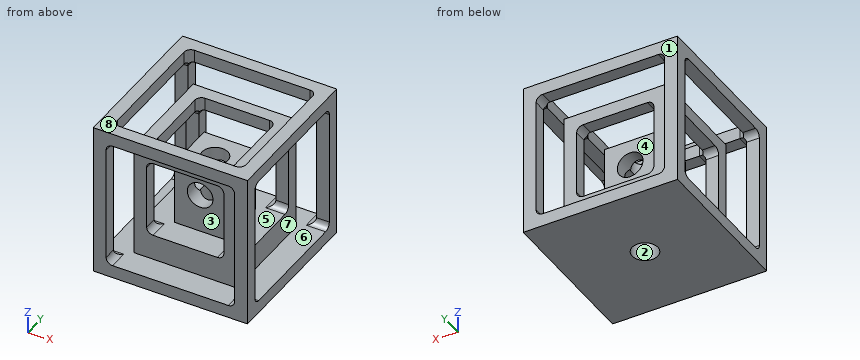
from build123d import *

# Parameters (mm, degrees)
SKETCH1_W           = 152.4
SKETCH1_H           = 152.4
EXTRUDE2_DEPTH      = 152.4
CUT_EXTRUDE14_DEPTH = 25.4
CUT_EXTRUDE18_DEPTH = 25.4
CUT_EXTRUDE19_DEPTH = 25.4
CUT_EXTRUDE21_START = -25.4
CUT_EXTRUDE21_DEPTH = 25.4
CUT_EXTRUDE22_START = -25.4
CUT_EXTRUDE22_DEPTH = 25.4
CUT_EXTRUDE24_DEPTH = 25.4
CUT_EXTRUDE27_DEPTH = 25.4
CUT_EXTRUDE28_START = -25.4
CUT_EXTRUDE28_DEPTH = 25.4
CUT_EXTRUDE29_DEPTH = 25.4
CUT_EXTRUDE30_START = -25.4
CUT_EXTRUDE30_DEPTH = 25.4
SKETCH30_R          = 12.7
CUT_EXTRUDE31_DEPTH = 239.273120599
SKETCH31_R          = 12.7
CUT_EXTRUDE32_DEPTH = 239.273120599
SKETCH32_R          = 12.7
CUT_EXTRUDE33_DEPTH = 239.273120599
SCALE1_SCALE        = 2


with BuildPart() as part:
    # Sketch1 → Extrude2 (new body)
    with BuildSketch(Plane(origin=(0, 0, 0), x_dir=(1, 0, 0), z_dir=(0, 1, 0))):
        with Locations((76.2, 76.2)):
            Rectangle(SKETCH1_W, SKETCH1_H)
    extrude(amount=EXTRUDE2_DEPTH)

    # Sketch13 → Cut-Extrude14 (cut)
    with BuildSketch(Plane(origin=(0, 152.4, 0), x_dir=(1, 0, 0), z_dir=(0, 1, 0))):
        with BuildLine():
            Line((19.05, 12.7), (133.35, 12.7))
            ThreePointArc((133.35, 12.7), (137.840128061, 14.559871939), (139.7, 19.05))
            Line((139.7, 19.05), (139.7, 133.35))
            ThreePointArc((139.7, 133.35), (137.840128061, 137.840128061), (133.35, 139.7))
            Line((133.35, 139.7), (19.05, 139.7))
            ThreePointArc((19.05, 139.7), (14.559871939, 137.840128061), (12.7, 133.35))
            Line((12.7, 133.35), (12.7, 19.05))
            ThreePointArc((12.7, 19.05), (14.559871939, 14.559871939), (19.05, 12.7))
        make_face()
    extrude(amount=-CUT_EXTRUDE14_DEPTH, mode=Mode.SUBTRACT)

    # Sketch17 → Cut-Extrude18 (cut)
    with BuildSketch(Plane.XY):
        with BuildLine():
            Line((19.05, 12.7), (133.35, 12.7))
            ThreePointArc((133.35, 12.7), (137.840128061, 14.559871939), (139.7, 19.05))
            Line((139.7, 19.05), (139.7, 133.35))
            ThreePointArc((139.7, 133.35), (137.840128061, 137.840128061), (133.35, 139.7))
            Line((133.35, 139.7), (19.05, 139.7))
            ThreePointArc((19.05, 139.7), (14.559871939, 137.840128061), (12.7, 133.35))
            Line((12.7, 133.35), (12.7, 19.05))
            ThreePointArc((12.7, 19.05), (14.559871939, 14.559871939), (19.05, 12.7))
        make_face()
    extrude(amount=-CUT_EXTRUDE18_DEPTH, mode=Mode.SUBTRACT)

    # Sketch18 → Cut-Extrude19 (cut)
    with BuildSketch(Plane(origin=(152.4, 0, 0), x_dir=(0, 0, -1), z_dir=(1, 0, 0))):
        with BuildLine():
            Line((19.05, 12.7), (133.35, 12.7))
            ThreePointArc((133.35, 12.7), (137.840128061, 14.559871939), (139.7, 19.05))
            Line((139.7, 19.05), (139.7, 133.35))
            ThreePointArc((139.7, 133.35), (137.840128061, 137.840128061), (133.35, 139.7))
            Line((133.35, 139.7), (19.05, 139.7))
            ThreePointArc((19.05, 139.7), (14.559871939, 137.840128061), (12.7, 133.35))
            Line((12.7, 133.35), (12.7, 19.05))
            ThreePointArc((12.7, 19.05), (14.559871939, 14.559871939), (19.05, 12.7))
        make_face()
    extrude(amount=-CUT_EXTRUDE19_DEPTH, mode=Mode.SUBTRACT)

    # Sketch20 → Cut-Extrude21 (cut)
    with BuildSketch(Plane.ZY.offset(CUT_EXTRUDE21_START)):
        with BuildLine():
            Line((-133.35, 12.7), (-19.05, 12.7))
            ThreePointArc((-19.05, 12.7), (-14.559871939, 14.559871939), (-12.7, 19.05))
            Line((-12.7, 19.05), (-12.7, 133.35))
            ThreePointArc((-12.7, 133.35), (-14.559871939, 137.840128061), (-19.05, 139.7))
            Line((-19.05, 139.7), (-133.35, 139.7))
            ThreePointArc((-133.35, 139.7), (-137.840128061, 137.840128061), (-139.7, 133.35))
            Line((-139.7, 133.35), (-139.7, 19.05))
            ThreePointArc((-139.7, 19.05), (-137.840128061, 14.559871939), (-133.35, 12.7))
        make_face()
    extrude(amount=CUT_EXTRUDE21_DEPTH, mode=Mode.SUBTRACT)

    # Sketch21 → Cut-Extrude22 (cut)
    with BuildSketch(Plane.XZ.offset(CUT_EXTRUDE22_START)):
        with BuildLine():
            Line((19.05, -139.7), (133.35, -139.7))
            ThreePointArc((133.35, -139.7), (137.840128061, -137.840128061), (139.7, -133.35))
            Line((139.7, -133.35), (139.7, -19.05))
            ThreePointArc((139.7, -19.05), (137.840128061, -14.559871939), (133.35, -12.7))
            Line((133.35, -12.7), (19.05, -12.7))
            ThreePointArc((19.05, -12.7), (14.559871939, -14.559871939), (12.7, -19.05))
            Line((12.7, -19.05), (12.7, -133.35))
            ThreePointArc((12.7, -133.35), (14.559871939, -137.840128061), (19.05, -139.7))
        make_face()
    extrude(amount=CUT_EXTRUDE22_DEPTH, mode=Mode.SUBTRACT)

    # Sketch23 → Cut-Extrude24 (cut)
    with BuildSketch(Plane.XY.offset(-25.4)):
        with BuildLine():
            Line((44.45, 38.1), (107.95, 38.1))
            ThreePointArc((107.95, 38.1), (112.440128061, 39.959871939), (114.3, 44.45))
            Line((114.3, 44.45), (114.3, 107.95))
            ThreePointArc((114.3, 107.95), (112.440128061, 112.440128061), (107.95, 114.3))
            Line((107.95, 114.3), (44.45, 114.3))
            ThreePointArc((44.45, 114.3), (39.959871939, 112.440128061), (38.1, 107.95))
            Line((38.1, 107.95), (38.1, 44.45))
            ThreePointArc((38.1, 44.45), (39.959871939, 39.959871939), (44.45, 38.1))
        make_face()
    extrude(amount=-CUT_EXTRUDE24_DEPTH, mode=Mode.SUBTRACT)

    # Sketch26 → Cut-Extrude27 (cut)
    with BuildSketch(Plane.XZ.offset(-25.4)):
        with BuildLine():
            Line((44.45, -114.3), (107.95, -114.3))
            ThreePointArc((107.95, -114.3), (112.440128061, -112.440128061), (114.3, -107.95))
            Line((114.3, -107.95), (114.3, -44.45))
            ThreePointArc((114.3, -44.45), (112.440128061, -39.959871939), (107.95, -38.1))
            Line((107.95, -38.1), (44.45, -38.1))
            ThreePointArc((44.45, -38.1), (39.959871939, -39.959871939), (38.1, -44.45))
            Line((38.1, -44.45), (38.1, -107.95))
            ThreePointArc((38.1, -107.95), (39.959871939, -112.440128061), (44.45, -114.3))
        make_face()
    extrude(amount=-CUT_EXTRUDE27_DEPTH, mode=Mode.SUBTRACT)

    # Sketch27 → Cut-Extrude28 (cut)
    with BuildSketch(Plane(origin=(0, 127, 0), x_dir=(-1, 0, 0), z_dir=(0, 1, 0)).offset(CUT_EXTRUDE28_START)):
        with BuildLine():
            Line((-107.95, -114.3), (-44.45, -114.3))
            ThreePointArc((-44.45, -114.3), (-39.959871939, -112.440128061), (-38.1, -107.95))
            Line((-38.1, -107.95), (-38.1, -44.45))
            ThreePointArc((-38.1, -44.45), (-39.959871939, -39.959871939), (-44.45, -38.1))
            Line((-44.45, -38.1), (-107.95, -38.1))
            ThreePointArc((-107.95, -38.1), (-112.440128061, -39.959871939), (-114.3, -44.45))
            Line((-114.3, -44.45), (-114.3, -107.95))
            ThreePointArc((-114.3, -107.95), (-112.440128061, -112.440128061), (-107.95, -114.3))
        make_face()
    extrude(amount=CUT_EXTRUDE28_DEPTH, mode=Mode.SUBTRACT)

    # Sketch28 → Cut-Extrude29 (cut)
    with BuildSketch(Plane(origin=(25.4, 0, 0), x_dir=(0, -1, 0), z_dir=(-1, 0, 0))):
        with BuildLine():
            Line((-107.95, -114.3), (-44.45, -114.3))
            ThreePointArc((-44.45, -114.3), (-39.959871939, -112.440128061), (-38.1, -107.95))
            Line((-38.1, -107.95), (-38.1, -44.45))
            ThreePointArc((-38.1, -44.45), (-39.959871939, -39.959871939), (-44.45, -38.1))
            Line((-44.45, -38.1), (-107.95, -38.1))
            ThreePointArc((-107.95, -38.1), (-112.440128061, -39.959871939), (-114.3, -44.45))
            Line((-114.3, -44.45), (-114.3, -107.95))
            ThreePointArc((-114.3, -107.95), (-112.440128061, -112.440128061), (-107.95, -114.3))
        make_face()
    extrude(amount=-CUT_EXTRUDE29_DEPTH, mode=Mode.SUBTRACT)

    # Sketch29 → Cut-Extrude30 (cut)
    with BuildSketch(Plane.YZ.offset(127).offset(CUT_EXTRUDE30_START)):
        with BuildLine():
            Line((44.45, -114.3), (107.95, -114.3))
            ThreePointArc((107.95, -114.3), (112.440128061, -112.440128061), (114.3, -107.95))
            Line((114.3, -107.95), (114.3, -44.45))
            ThreePointArc((114.3, -44.45), (112.440128061, -39.959871939), (107.95, -38.1))
            Line((107.95, -38.1), (44.45, -38.1))
            ThreePointArc((44.45, -38.1), (39.959871939, -39.959871939), (38.1, -44.45))
            Line((38.1, -44.45), (38.1, -107.95))
            ThreePointArc((38.1, -107.95), (39.959871939, -112.440128061), (44.45, -114.3))
        make_face()
    extrude(amount=CUT_EXTRUDE30_DEPTH, mode=Mode.SUBTRACT)

    # Sketch30 → Cut-Extrude31 (cut, through all)
    with BuildSketch(Plane.XY.offset(-50.8)):
        with Locations((76.2, 76.2)):
            Circle(SKETCH30_R)
    extrude(amount=-CUT_EXTRUDE31_DEPTH, mode=Mode.SUBTRACT)

    # Sketch31 → Cut-Extrude32 (cut, through all)
    with BuildSketch(Plane(origin=(101.6, 0, 0), x_dir=(0, 0, -1), z_dir=(1, 0, 0))):
        with Locations((76.2, 76.2)):
            Circle(SKETCH31_R)
    extrude(amount=-CUT_EXTRUDE32_DEPTH, mode=Mode.SUBTRACT)

    # Sketch32 → Cut-Extrude33 (cut, through all)
    with BuildSketch(Plane.XZ.offset(-50.8)):
        with Locations(Location((76.2, -76.2, 0), (0, 0, 225))):
            Circle(SKETCH32_R)
    extrude(amount=-CUT_EXTRUDE33_DEPTH, mode=Mode.SUBTRACT)


with BuildPart() as part_1:
    # Scale1: scaled about (76.199999991, 76.199999991, -102.985994001)
    add(part.part.scale(SCALE1_SCALE).moved(Location((-76.199999991, -76.199999991, 102.985994001))))


solid = part_1.part
Can you work these out from the model? Positions are in its coordinate system, mm. Face numbers are marked on the shaded views. A direction names the side the tool comes from. Give positions to 0.01 mm unless a question says otherwise; leave off trailing zeros. Loops run counter-clockwise (first coordinate to the right, second up) from the corner with the lowest first, then second, coordinate; pieces in that order, holes last. Notation, with made-up numbers: (77, 81) - (106, 81) arc R23 cw to (106, 119) - close; hole circle Ø7 at (88, 5.5). An arc over 180 degrees is marked (long way). Return JSON: item names as keys, results as strings.
1. I want a section at A-A on z = 35. Please give me the cut outline in (x, y).
Output values:
{"outline": "(-76.2, -76.2) - (-50.8, -76.2) - (-50.8, -50.8) - (-76.2, -50.8) - close; (-76.2, 203.2) - (-50.8, 203.2) - (-50.8, 228.6) - (-76.2, 228.6) - close; (-25.4, -25.4) - (177.8, -25.4) - (177.8, 177.8) - (-25.4, 177.8) - close; (203.2, -76.2) - (228.6, -76.2) - (228.6, -50.8) - (203.2, -50.8) - close; (203.2, 203.2) - (228.6, 203.2) - (228.6, 228.6) - (203.2, 228.6) - close; hole (0, 12.7) arc R12.7 ccw to (12.7, 0) - (139.7, 0) arc R12.7 ccw to (152.4, 12.7) - (152.4, 139.7) arc R12.7 ccw to (139.7, 152.4) - (12.7, 152.4) arc R12.7 ccw to (0, 139.7) - close"}
2. I want a section at C-C on y = 120. Give the number of separate pieces and of enclosed holes in the cut face, and give its area (3 significant figures).
Output values:
{"separate pieces": "5", "enclosed holes": "1", "area": "31,500 mm²"}
3. I want a section at B-B on y = -11. Please give me the cut outline in (x, z).
Output values:
{"outline": "(-76.2, -201.81) - (228.6, -201.81) - (228.6, -176.41) - (177.8, -176.41) - (177.8, 52.19) - (-25.4, 52.19) - (-25.4, -176.41) - (-76.2, -176.41) - close; (-76.2, 77.59) - (-50.8, 77.59) - (-50.8, 102.99) - (-76.2, 102.99) - close; (203.2, 77.59) - (228.6, 77.59) - (228.6, 102.99) - (203.2, 102.99) - close; hole (0, -112.91) arc R12.7 ccw to (12.7, -125.61) - (139.7, -125.61) arc R12.7 ccw to (152.4, -112.91) - (152.4, 14.09) arc R12.7 ccw to (139.7, 26.79) - (12.7, 26.79) arc R12.7 ccw to (0, 14.09) - close"}
4. For the marked faces 1, 2, 3, 4 and 5, which set-ups out of +Z, -Z, +X, -X, +Y, -Y let a thin tool reach every point of the face, with its end or its side?
Output values:
{"face 1": "+Z, -Z, +X, -X, +Y", "face 2": "+Z, -Z", "face 3": "+Z, +X, -X, -Y", "face 4": "+Z, +X, -X, +Y", "face 5": "none"}
5. We'd pull the mould along Z, two halves only. Please class the marked faces 6, 7 and 8: +Z half, -Z half, draft (parallel to the pull), parting line (faces both ways), or undercut.
Output values:
{"face 6": "undercut", "face 7": "draft", "face 8": "+Z half"}
6. If I drill on line 1 (Y direction, x = -5, z = -114); line 2 (Z direction, x = 156, y = 100); line 3 (X direction, y = 76, z = -144), over which ranges is the centre line in solid material (lowest first)?
Output values:
{"line 1": "y = -25.4 to 0.05, 152.35 to 177.8", "line 2": "z = -201.81 to -125.61, 26.79 to 52.19", "line 3": "x = -25.4 to 50.8, 101.6 to 177.8"}
7. I'm going to push flat-ended pins straight in: pin 1 Ø8 at (x, z) = (22, 6) entering from -Y; pin 2 Ø1 at (y, z) = (177.5, -34.5) entering from +X; pin 3 Ø2 at (x, y) = (168.5, -30.5) entering from +Z; pin 4 Ø20.5 at (x, z) = (164, -43.5) entering from -Y. Where does each tip first touch, or does it pass through?
Output values:
{"pin 1": "passes through", "pin 2": "stops at x = 177.8", "pin 3": "stops at z = -176.41", "pin 4": "stops at y = -25.4"}
